The listing builds one solid part. Answer for the finished solid, in the listing's coordinates (mm). Face numbers are marked on the shaded views. A direction names the side the tool comes from. Coordinates: 2 decimals unless noted, no trailing zeros. Use a Markdown table: item, result. Add a question column.
Item 1: A flat-ended cylindrical pin translates along its axis: P1, Ø3, axis at x = -4.33, y = 0, coming from the +Z side. Find the tip coordinate at first contact, or state that the pin passes through.
Item 2: Find the intervals of material crossed by line 1 along X through (y, z) = (0, 8); line 2 along Y through (x, z) = (4.25, 5.25); line 3 along X through (y, z) = (5.25, 8.25), in increasing order.
Item 3: The mould has two halves that part along Y. Classify the marked faces 1, 2 and 3: released by +Y, released by -Y, zero draft, split by the parting line, or undercut.
Item 4: The part is cut by section A-A, the plane z = 6. State how many separate pieces and enclosed holes the cut face has, then the cut area to 3 significant figures.
Item 5: For the marked faces 4 and 5, determine the directions among +Z, -Z, +X, -X, +Y, -Y from which every point of the face is accessible in a straight line to the end or side of a thin tool.
from build123d import *

# Parameters (mm, degrees)
F0_W           = 15
F0_H           = 15
F1_DEPTH       = 15
F2_R           = 2.1
F3_DEPTH       = 10
F4_DEPTH       = 10
F6_D           = 3.6
F6_DEPTH       = 10
F6_TIP         = 1.0815491142
F9_R           = 2.1
F10_DEPTH      = 10
F10_DEPTH_BACK = 10
F11_DEPTH      = 10
F11_DEPTH_BACK = 10


with BuildPart() as f1:
    # F0 (on Top) → F1 (new body)
    with BuildSketch(Plane.XY):
        Rectangle(F0_W, F0_H)
    extrude(amount=F1_DEPTH)

    # F2 (on face) → F3 (cut)
    with BuildSketch(Plane.XY.offset(15)):
        with Locations((-3.3081052825, 4.5566549525)):
            Circle(F2_R)
    extrude(amount=-F3_DEPTH, mode=Mode.SUBTRACT)

    # F2 (on face) → F4 (cut)
    with BuildSketch(Plane.XY.offset(15)):
        with BuildLine():
            ThreePointArc((3.2809909909, 5.6586071096), (4.271900841, 5.899439318), (5.2151213678, 5.5118344659))
            ThreePointArc((5.2151213678, 5.5118344659), (5.0605091693, 5.7942622045), (5.1341789855, 6.1076997863))
            ThreePointArc((5.1341789855, 6.1076997863), (4.3059514618, 6.3481491967), (3.450923876, 6.2354346119))
            ThreePointArc((3.450923876, 6.2354346119), (3.4764516514, 5.9144693594), (3.2809909909, 5.6586071096))
        make_face()
        with BuildLine():
            ThreePointArc((3.5456670252, 2.2421209971), (3.7136732609, 2.5167921893), (4.0221963108, 2.608900206))
            ThreePointArc((4.0221963108, 2.608900206), (3.0789758, 2.9965050415), (2.5437227765, 3.8644950423))
            ThreePointArc((2.5437227765, 3.8644950423), (2.5027997945, 3.5451274527), (2.2589656824, 3.334853171))
            ThreePointArc((2.2589656824, 3.334853171), (2.787683207, 2.6535055877), (3.5456670252, 2.2421209971))
        make_face()
        with BuildLine():
            ThreePointArc((5.8747835443, 3.0604646595), (5.6654725032, 3.3051261397), (5.6732114262, 3.6270119283))
            ThreePointArc((5.6732114262, 3.6270119283), (5.0131061422, 2.8497324056), (4.0221963108, 2.608900206))
            ThreePointArc((4.0221963108, 2.608900206), (4.313287058, 2.471290132), (4.4379209082, 2.174411775))
            ThreePointArc((4.4379209082, 2.174411775), (5.2493036675, 2.4667040397), (5.8747835443, 3.0604646595))
        make_face()
        with BuildLine():
            ThreePointArc((5.2151213678, 5.5118344659), (5.644516455, 4.9470549944), (5.7970485739, 4.2541697621))
            ThreePointArc((5.7970485739, 4.2541697621), (5.7657932583, 3.9345361486), (5.6732114262, 3.6270119283))
            ThreePointArc((5.6732114262, 3.6270119283), (5.8940383698, 3.8613318458), (6.2149004544, 3.8881252289))
            ThreePointArc((6.2149004544, 3.8881252289), (6.1876450529, 4.7501193664), (5.816229058, 5.5284682012))
            ThreePointArc((5.816229058, 5.5284682012), (5.5188614887, 5.4050061266), (5.2151213678, 5.5118344659))
        make_face()
        with BuildLine():
            ThreePointArc((2.5437227765, 3.8644950423), (2.6208857067, 4.8813275594), (3.2809909909, 5.6586071096))
            ThreePointArc((3.2809909909, 5.6586071096), (2.9646084595, 5.598837153), (2.6892768391, 5.7657588495))
            ThreePointArc((2.6892768391, 5.7657588495), (2.2046594805, 5.0523706202), (2.0476393662, 4.204360341))
            ThreePointArc((2.0476393662, 4.204360341), (2.360783986, 4.1294549747), (2.5437227765, 3.8644950423))
        make_face()
        with BuildLine():
            ThreePointArc((5.6732114262, 3.6270119283), (5.7657932583, 3.9345361486), (5.7970485739, 4.2541697621))
            ThreePointArc((5.7970485739, 4.2541697621), (5.644516455, 4.9470549944), (5.2151213678, 5.5118344659))
            ThreePointArc((5.2151213678, 5.5118344659), (4.271900841, 5.899439318), (3.2809909909, 5.6586071096))
            ThreePointArc((3.2809909909, 5.6586071096), (2.6208857067, 4.8813275594), (2.5437227765, 3.8644950423))
            ThreePointArc((2.5437227765, 3.8644950423), (3.0789758, 2.9965050415), (4.0221963108, 2.608900206))
            ThreePointArc((4.0221963108, 2.608900206), (5.0131061422, 2.8497324056), (5.6732114262, 3.6270119283))
        make_face()
    extrude(amount=-F4_DEPTH, mode=Mode.SUBTRACT)

    # F6
    with Locations(Plane.XY.offset(15)):
        with Locations((-4.327217117, 0)):
            Hole(F6_D / 2, depth=F6_DEPTH)
            with Locations((0, 0, -(F6_DEPTH + F6_TIP / 2))):  # 118° drill point
                Cone(0, F6_D / 2, F6_TIP, mode=Mode.SUBTRACT)

    # F9 (on line) → F10 (cut, two sides)
    with BuildSketch(Plane(origin=(0, -6.5801176454, 13.4912404864), x_dir=(1, 0, 0), z_dir=(0, -0.4383711468, 0.8987940463))) as f10_sk:
        with Locations((-1.1891657487, 0)):
            Circle(F9_R)
    extrude(amount=-F10_DEPTH, mode=Mode.SUBTRACT)
    extrude(f10_sk.sketch, amount=F10_DEPTH_BACK, mode=Mode.SUBTRACT)

    # F9 (on line) → F11 (cut, two sides)
    with BuildSketch(Plane(origin=(0, -6.5801176454, 13.4912404864), x_dir=(1, 0, 0), z_dir=(0, -0.4383711468, 0.8987940463))) as f11_sk:
        with BuildLine():
            ThreePointArc((4.9336170518, -1.6870876514), (4.9217202173, -1.3653287012), (5.1278529304, -1.117983474))
            ThreePointArc((5.1278529304, -1.117983474), (4.1276234932, -1.3165874448), (3.2016843949, -0.8893413207))
            ThreePointArc((3.2016843949, -0.8893413207), (3.3441834561, -1.178070216), (3.2572910424, -1.4881025786))
            ThreePointArc((3.2572910424, -1.4881025786), (4.0745795038, -1.7634502148), (4.9336170518, -1.6870876514))
        make_face()
        with BuildLine():
            ThreePointArc((2.6004119701, -0.8804748841), (2.9027465931, -0.7697313384), (3.2016843949, -0.8893413207))
            ThreePointArc((3.2016843949, -0.8893413207), (2.7037129005, 0.0005613942), (2.823917186, 1.0132081149))
            ThreePointArc((2.823917186, 1.0132081149), (2.5933543197, 0.7884613294), (2.2716447953, 0.7752956598))
            ThreePointArc((2.2716447953, 0.7752956598), (2.2623296555, -0.0870789562), (2.6004119701, -0.8804748841))
        make_face()
        with BuildLine():
            ThreePointArc((5.1278529304, -1.117983474), (5.7454877945, -0.5126676326), (5.9721181259, 0.3219093778))
            ThreePointArc((5.9721181259, 0.3219093778), (5.9642004358, 0.483358092), (5.9405233533, 0.6432573507))
            ThreePointArc((5.9405233533, 0.6432573507), (5.4425518562, 1.5331600768), (4.5166127528, 1.9604062012))
            ThreePointArc((4.5166127528, 1.9604062012), (3.5163833114, 1.7618022241), (2.823917186, 1.0132081149))
            ThreePointArc((2.823917186, 1.0132081149), (2.7037129005, 0.0005613942), (3.2016843949, -0.8893413207))
            ThreePointArc((3.2016843949, -0.8893413207), (4.1276234932, -1.3165874448), (5.1278529304, -1.117983474))
        make_face()
        with BuildLine():
            ThreePointArc((5.9405233533, 0.6432573507), (5.9642004358, 0.483358092), (5.9721181259, 0.3219093778))
            ThreePointArc((5.9721181259, 0.3219093778), (5.7454877945, -0.5126676326), (5.1278529304, -1.117983474))
            ThreePointArc((5.1278529304, -1.117983474), (5.4464850598, -1.0716809479), (5.7144921267, -1.2501258132))
            ThreePointArc((5.7144921267, -1.2501258132), (6.2289193143, -0.5579253952), (6.4217514019, 0.2826651924))
            ThreePointArc((6.4217514019, 0.2826651924), (6.1120641324, 0.3707796135), (5.9405233533, 0.6432573507))
        make_face()
        with BuildLine():
            ThreePointArc((4.5166127528, 1.9604062012), (5.4425518562, 1.5331600768), (5.9405233533, 0.6432573507))
            ThreePointArc((5.9405233533, 0.6432573507), (5.9949497762, 0.9606027823), (6.2474796669, 1.1603501546))
            ThreePointArc((6.2474796669, 1.1603501546), (5.7481246921, 1.8635011762), (5.0082639284, 2.3066521666))
            ThreePointArc((5.0082639284, 2.3066521666), (4.8287635013, 2.039350922), (4.5166127528, 1.9604062012))
        make_face()
        with BuildLine():
            ThreePointArc((2.823917186, 1.0132081149), (3.5163833114, 1.7618022241), (4.5166127528, 1.9604062012))
            ThreePointArc((4.5166127528, 1.9604062012), (4.2316180075, 2.1102339389), (4.119682998, 2.4121294665))
            ThreePointArc((4.119682998, 2.4121294665), (3.2966374636, 2.1545002791), (2.646546277, 1.5877920657))
            ThreePointArc((2.646546277, 1.5877920657), (2.8452961865, 1.3344763829), (2.823917186, 1.0132081149))
        make_face()
    extrude(amount=-F11_DEPTH, mode=Mode.SUBTRACT)
    extrude(f11_sk.sketch, amount=F11_DEPTH_BACK, mode=Mode.SUBTRACT)


solid = f1.part
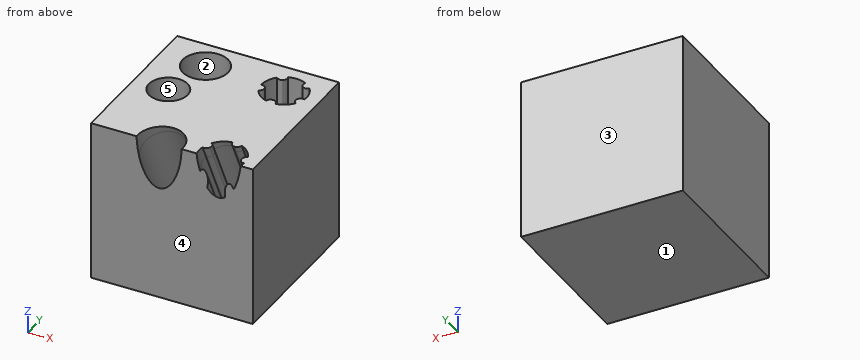
Solution:
| question | item | result |
|---|---|---|
| 1 | P1 | stops at z = 4.82 |
| 2 | line 1 | x = -7.5 to -6.13, -2.53 to 7.5 |
| 2 | line 2 | y = -7.5 to -4.54, -0.67 to 2.53, 6.35 to 7.5 |
| 2 | line 3 | x = -7.5 to -5.29, -1.33 to 2.3, 6 to 7.5 |
| 3 | face 1 | zero draft |
| 3 | face 2 | undercut |
| 3 | face 3 | released by +Y |
| 4 | separate pieces | 1 |
| 4 | enclosed holes | 5 |
| 4 | area | 159 mm2 |
| 5 | face 4 | +Z, -Z, +X, -X, -Y |
| 5 | face 5 | +Z |
